Work out the finished part from the listing and answer in its coordinate system (mm). A direction names the side the tool comes from. Round coordinates to 2 decimals unless told otherwise and drop trailing zeros. Write each loop counter-clockwise with the first axis right and the second up, starting at its lowest first coordinate (ties: lowest second). Pieces come first, ordered by that corner, then holes. Notation, with made-up numbers: (-37, 74.5) - (-19, 74.5) arc R12 ccw to (-19, 90.5) - close; hole circle Ø9 at (81, 32). An arc over 180 degrees is marked (long way). Answer as a JSON object with one key per item and string values.
```python
from build123d import *

# Parameters (mm, degrees)
SKETCH4_W           = 57.15
SKETCH4_H           = 10.16
BOSS_EXTRUDE1_DEPTH = 12.7
SKETCH5_R           = 10
CUT_EXTRUDE1_DEPTH  = 60.419172832
SKETCH8_R           = 1.5875
CUT_EXTRUDE3_DEPTH  = 60.419172832
SKETCH9_W           = 6.35
SKETCH9_H           = 6.35
BOSS_EXTRUDE2_DEPTH = 28.575
SKETCH11_W          = 57.15
SKETCH11_H          = 10.16
BOSS_EXTRUDE3_DEPTH = 12.7


with BuildPart() as part:
    # Sketch4 → Boss-Extrude1 (new body)
    with BuildSketch(Plane.XY):
        with Locations((28.575, 5.08)):
            Rectangle(SKETCH4_W, SKETCH4_H)
    extrude(amount=BOSS_EXTRUDE1_DEPTH)

    # Sketch5 → Cut-Extrude1 (cut, through all)
    with BuildSketch(Plane.XY.offset(12.7)):
        with Locations((15.875, 16.5)):
            Circle(SKETCH5_R)
        with Locations((41.275, 16.5)):
            Circle(SKETCH5_R)
    extrude(amount=-CUT_EXTRUDE1_DEPTH, mode=Mode.SUBTRACT)

    # Sketch8 → Cut-Extrude3 (cut, through all)
    with BuildSketch(Plane(origin=(0, 10.16, 0), x_dir=(1, 0, 0), z_dir=(0, 1, 0))):
        with Locations(Location((28.575, -6.35, 0), (0, 0, 270))):
            Circle(SKETCH8_R)
    extrude(amount=-CUT_EXTRUDE3_DEPTH, mode=Mode.SUBTRACT)

    # Sketch9 → Boss-Extrude2 (add)
    with BuildSketch(Plane(origin=(0, 0, 0), x_dir=(-1, 0, 0), z_dir=(0, 0, -1))):
        with Locations((-53.975, 3.175)):
            Rectangle(SKETCH9_W, SKETCH9_H)
        with Locations((-3.175, 3.175)):
            Rectangle(SKETCH9_W, SKETCH9_H)
    extrude(amount=BOSS_EXTRUDE2_DEPTH)

    # Sketch11 → Boss-Extrude3 (add)
    with BuildSketch(Plane(origin=(0, 0, -28.575), x_dir=(-1, 0, 0), z_dir=(0, 0, -1))):
        with Locations((-28.575, 5.08)):
            Rectangle(SKETCH11_W, SKETCH11_H)
    extrude(amount=BOSS_EXTRUDE3_DEPTH)


solid = part.part
```
Item 1: Consider line 1 along Z through (x, y) = (12.5, 1.75) (3 decimals); line 2 along X through (y, z) = (1.25, -5); line 3 along X through (y, z) = (8, 6.35). Determine where each line is inside the solid, lowest interval first.
Results found:
{"line 1": "-41.275 to -28.575, 0 to 12.7", "line 2": "0 to 6.35, 50.8 to 57.15", "line 3": "0 to 10.61, 21.14 to 26.99, 30.16 to 36.01, 46.54 to 57.15"}
Item 2: Determine the mould class of faces 6 (the flat face through (29, 5, -28.575)), 7 (the cylindrical face through (27.025, 5.151, 6.006)), 8 (the flat face through (4, 10.16, 6)), 9 (the flat face through (28, 4, 12.7)) for opening direction Z: pulls with the +Z half, pulls with the -Z half, needs draft (parallel to the pull), parting line crosses it, or undercut.
Results found:
{"face 6": "undercut", "face 7": "undercut", "face 8": "needs draft", "face 9": "pulls with the +Z half"}
Item 3: A cutting plane is placed at D-D (z = 9.5). Write down the section's boundary in (x, y) (3 decimals), and give its area (3 significant figures).
Results found:
{"outline": "(0, 0) - (57.15, 0) - (57.15, 10.16) - (49.008, 10.16) arc R10 cw to (33.542, 10.16) - (23.608, 10.16) arc R10 cw to (8.142, 10.16) - (0, 10.16) - close", "area": "502 mm²"}
Item 4: A cutting plane is placed at A-A (z = -24). Write down the section's boundary in (x, y).
Results found:
{"outline": "(0, 0) - (6.35, 0) - (6.35, 6.35) - (0, 6.35) - close; (50.8, 0) - (57.15, 0) - (57.15, 6.35) - (50.8, 6.35) - close"}
Item 5: For faces 1 (the flat face through (50.8, 3, -14)), 2 (the cylindrical face through (41.2, 6.5, 6.4)), 3 (the flat face through (29, 0, 4)), 4 (the flat face through (57.15, 4, -14)), 5 (the flat face through (3, 6.35, -14)), determine the directions among +Z, -Z, +X, -X, +Y, -Y from which every point of the face is accessible in a straight line to the end or side of a thin tool.
Results found:
{"face 1": "+Y, -Y", "face 2": "+Z, +Y", "face 3": "+Z, -Z, +X, -X, -Y", "face 4": "+Z, -Z, +X, +Y, -Y", "face 5": "+X, -X, +Y"}
Item 6: Each of these flat-tipped pins is pushed along its axis until it touches: P1, Ø5, axis at x = 55, z = -19, coming from the +Y side; P2, Ø2, axis at y = 7.5, z = 3, coming from the -X side. Where does it stop, or does it pass through?
Results found:
{"P1": "y = 6.35", "P2": "x = 0"}
Item 7: A cutting plane is placed at B-B (y = 7.25). Give the number of separate pieces and of enclosed holes in the cut face, and give its area (3 significant figures).
Results found:
{"separate pieces": "4", "enclosed holes": "1", "area": "1,250 mm²"}
Item 8: A cutting plane is placed at C-C (x = 41.5). Write down the section's boundary in (y, z) (3 decimals), and give its area (3 significant figures).
Results found:
{"outline": "(0, -41.275) - (10.16, -41.275) - (10.16, -28.575) - (0, -28.575) - close; (0, 0) - (6.503, 0) - (6.503, 12.7) - (0, 12.7) - close", "area": "212 mm²"}
